from build123d import *

# Parameters (mm, degrees)
SKETCH1_W                                 = 60
SKETCH1_H                                 = 60
BOSS_EXTRUDE1_DEPTH                       = 10
FILLET1_R                                 = 3
M3X0_5_TAPPED_HOLE1_OUTLINE_R             = 1.25
M3X0_5_TAPPED_HOLE1_DEPTH                 = 10
CSK_FOR_8_FLAT_HEAD_MACHINE_SCREW_2_COUNT = 2
CSK_FOR_8_FLAT_HEAD_MACHINE_SCREW_2_PITCH = 30
CHAMFER1_SIZE                             = 1


# Read off the part's stored shape, not the designer's step: M3x0.5 Tapped Hole1
with BuildPart() as part:
    # Sketch1 → Boss-Extrude1 (new body)
    with BuildSketch(Plane(origin=(0, 0, 0), x_dir=(1, 0, 0), z_dir=(0, 1, 0))):
        Rectangle(SKETCH1_W, SKETCH1_H)
    extrude(amount=BOSS_EXTRUDE1_DEPTH)

    # Fillet1
    fillet1_edges = [part.edges().sort_by_distance(p)[0] for p in [
        (30, 5, 30),
        (-30, 5, 30),
        (-30, 5, -30),
        (30, 5, -30),
    ]]
    fillet(fillet1_edges, radius=FILLET1_R)

    # M3x0.5 Tapped Hole1 outline → M3x0.5 Tapped Hole1 (cut)
    with BuildSketch(Plane(origin=(0, 0, 0), x_dir=(1, 0, 0), z_dir=(0, 1, 0))):
        with Locations((23, -23)):
            Circle(M3X0_5_TAPPED_HOLE1_OUTLINE_R)
        with Locations((-23, 23)):
            Circle(M3X0_5_TAPPED_HOLE1_OUTLINE_R)
        with Locations((-23, -23)):
            Circle(M3X0_5_TAPPED_HOLE1_OUTLINE_R)
        with Locations((23, 23)):
            Circle(M3X0_5_TAPPED_HOLE1_OUTLINE_R)
    extrude(amount=M3X0_5_TAPPED_HOLE1_DEPTH, mode=Mode.SUBTRACT)

    # Sketch7 → CSK for #8 Flat Head Machine Screw (100)2 (revolve, cut)
    with BuildSketch(Plane(origin=(15, 10, 0), x_dir=(0, 0, 1), z_dir=(1, 0, 0))):
        Polygon((0, 0), (0, 10), (2.2479, 10), (2.2479, 7.651767624), (4.2164, 6), (4.2164, 0), align=None)
    csk_for_8_flat_head_machine_screw_100 = revolve(axis=Axis((15, 16.35, 0), (0, -1, 0)), mode=Mode.SUBTRACT)

    # CSK for _8 Flat Head Machine Screw _ 2: CSK for #8 Flat Head Machine Screw (100)2 ×2
    with Locations(*[(-i * CSK_FOR_8_FLAT_HEAD_MACHINE_SCREW_2_PITCH, 0, 0) for i in range(1, CSK_FOR_8_FLAT_HEAD_MACHINE_SCREW_2_COUNT)]):
        add(csk_for_8_flat_head_machine_screw_100, mode=Mode.SUBTRACT)

    # Chamfer1
    chamfer1_edges = [part.edges().sort_by_distance(p)[0] for p in [
        (-30, 0, 0),
        (-30, 10, 0),
        (30, 0, 0),
        (0, 0, 30),
        (0, 0, -30),
        (-29.121320344, 0, 29.121320344),
        (29.121320344, 0, 29.121320344),
        (29.121320344, 0, -29.121320344),
        (-29.121320344, 0, -29.121320344),
        (0, 10, -30),
        (30, 10, 0),
        (0, 10, 30),
        (-29.121320344, 10, 29.121320344),
        (29.121320344, 10, 29.121320344),
        (29.121320344, 10, -29.121320344),
        (-29.121320344, 10, -29.121320344),
    ]]
    chamfer(chamfer1_edges, length=CHAMFER1_SIZE)


solid = part.part
Geometry check sheet. Reference: the model listing, model coordinates, mm. A direction names the side the tool comes from. Round coordinates to 2 decimals unless told otherwise and drop trailing zeros. Write each loop counter-clockwise with the first axis right and the second up, starting at its lowest first coordinate (ties: lowest second). Pieces come first, ordered by that corner, then holes.
Item 1: Go/stop test with flat-tipped pins: pin 1 Ø2 at (x, z) = (23, 23) entering from +Y; pin 2 Ø6.5 at (x, z) = (15, 0) entering from +Y. Record where each tip stops, or that it passes through.
Determined:
pin 1: passes through
pin 2: stops at y = 3.19
Item 2: Mould release check, pull along X, two halves, no side actions. Record for faces 3 (the face through (-29.14, 5.06, -29.1)), 4 (the face through (28.666, 9.618, -28.703)), 5 (the face through (12.65, 2.45, -0.31)), 6 (the face through (17.194, 1.191, -0.487)): +X half, -X half, draft (parallel to the pull), parting line (faces both ways), or undercut.
Determined:
face 3: -X half
face 4: +X half
face 5: undercut
face 6: undercut
Item 3: Access from +Z, -Z, +X, -X, +Y, -Y to the whole of each face (thin tool, end or side, straight path). Record for faces 1 (the face through (24.155, 4.93, -22.521)), 2 (the face through (-10.884, 7.042, -0.914)).
Determined:
face 1: +Y, -Y
face 2: +Y
Item 4: Section check B-B (z = 0). Record the boundary of the cut face in (x, y), plus the area to 3 significant figures.
Determined:
outline: (-30, 1) - (-29, 0) - (-17.25, 0) - (-17.25, 2.35) - (-19.22, 4) - (-19.22, 10) - (-29, 10) - (-30, 9) - close; (-12.75, 0) - (12.75, 0) - (12.75, 2.35) - (10.78, 4) - (10.78, 10) - (-10.78, 10) - (-10.78, 4) - (-12.75, 2.35) - close; (17.25, 0) - (29, 0) - (30, 1) - (30, 9) - (29, 10) - (19.22, 10) - (19.22, 4) - (17.25, 2.35) - close
area: 454 mm2
Item 5: Material ranges on line 1 along Z through (x, y) = (23, 4.5); line 2 along X through (y, z) = (7.55, 0), recorded low to high.
Determined:
line 1: z = -30 to -24.25, -21.75 to 21.75, 24.25 to 30
line 2: x = -30 to -19.22, -10.78 to 10.78, 19.22 to 30
Item 6: Section check C-C (x = 15). Record the boundary of the cut face in (y, z), plus the area to 3 significant figures.
Determined:
outline: (0, -29) - (1, -30) - (9, -30) - (10, -29) - (10, -4.22) - (4, -4.22) - (2.35, -2.25) - (0, -2.25) - close; (0, 2.25) - (2.35, 2.25) - (4, 4.22) - (10, 4.22) - (10, 29) - (9, 30) - (1, 30) - (0, 29) - close
area: 526 mm2
Item 7: Section check D-D (y = 6). Record the boundary of the cut face in (x, z).
Determined:
outline: (-30, -27) arc R3 ccw to (-27, -30) - (27, -30) arc R3 ccw to (30, -27) - (30, 27) arc R3 ccw to (27, 30) - (-27, 30) arc R3 ccw to (-30, 27) - close; hole circle Ø2.5 at (-23, -23); hole circle Ø2.5 at (-23, 23); hole circle Ø8.43 at (-15, 0); hole circle Ø8.43 at (15, 0); hole circle Ø2.5 at (23, -23); hole circle Ø2.5 at (23, 23)
Item 8: Section check A-A (x = -23). Record the boundary of the cut face in (y, z), plus the area to 3 significant figures.
Determined:
outline: (0, -29) - (1, -30) - (9, -30) - (10, -29) - (10, -24.25) - (0, -24.25) - close; (0, -21.75) - (10, -21.75) - (10, 21.75) - (0, 21.75) - close; (0, 24.25) - (10, 24.25) - (10, 29) - (9, 30) - (1, 30) - (0, 29) - close
area: 548 mm2
